Input: part model. Units: mm. Frame: model coordinates. Give positions to 0.01 mm unless a question says otherwise; leave off trailing zeros. Order: outer loops, then holes, each group sorted by start corner. A loop starts at its lowest first (then second) coordinate and runs counter-clockwise, first axis right, second up. Notation, with made-up numbers: (-25.75, 31.25) - (-5.75, 31.25) arc R7 ccw to (-5.75, 42.25) - close; hole circle Ø1 at (88.5, 82.5). An arc over 180 degrees is marked (long way). Answer in a Markdown table with one row per item. Add a question column.
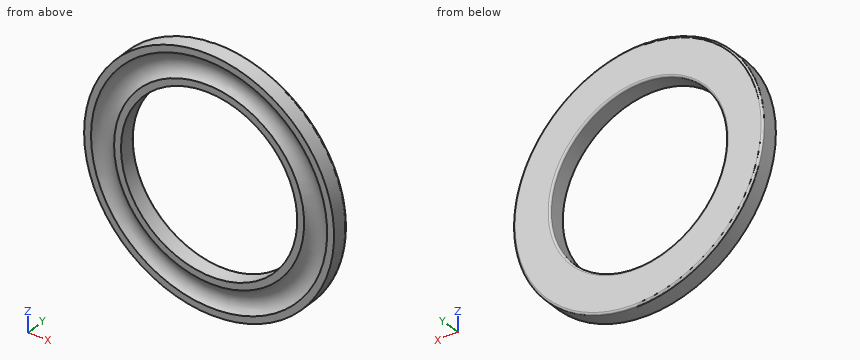
Autodesk Inventor part; units mm, degrees
ref_plane "tb_sdt_srd_XY" through (0, 0, 0) normal (0, 1, 0) x (1, 0, 0)
ref_plane "tb_sdt_srd_YZ" through (0, 0, 0) normal (1, 0, 0) x (0, 0, -1)
ref_plane "tb_sdt_srd_ZX" through (0, 0, 0) normal (0, 0, -1) x (0, 1, 0)
sketch "Sketch_1" plane through (0, 0, 0) normal (0, 0, 1) x (1, 0, 0)
  line L0 (0, 16) -> (0, 10.6667)
  line L1 (-39, 10.6667) -> (-36.8499, 10.6667)
  arc A0 (-29.6501, 10.6667) -> (-36.8499, 10.6667) centre (-33.25, 8) ccw
  line L2 (-29.6501, 10.6667) -> (-27.5, 10.6667)
  line L3 (-27.5, 10.6667) -> (-27.5, 15.4)
  arc A1 (-27.5, 15.4) -> (-28.1, 16) centre (-28.1, 15.4) ccw
  line L4 (-28.1, 16) -> (-38.4, 16)
  arc A2 (-38.4, 16) -> (-39, 15.4) centre (-38.4, 15.4) ccw
  line L5 (-39, 15.4) -> (-39, 10.6667)
revolve "Revolution1" add sketch "Sketch_1" angle 360 about axis through (0, 16, 0) along (0, 1, 0)
ref_plane "tb_sdt_srd_XY" through (0, 0, 0) normal (0, 1, 0) x (1, 0, 0)
ref_plane "tb_sdt_srd_YZ" through (0, 0, 0) normal (1, 0, 0) x (0, 0, -1)
ref_plane "tb_sdt_srd_ZX" through (0, 0, 0) normal (0, 0, -1) x (0, 1, 0)
ref_plane "tb_sdt_srd1_1_XY" through (0, 8, -33.25) normal (0, 1, 0) x (1, 0, 0)
ref_plane "tb_sdt_srd1_1_YZ" through (0, 8, -33.25) normal (1, 0, 0) x (0, 0, -1)
ref_plane "tb_sdt_srd1_1_ZX" through (0, 8, -33.25) normal (0, 0, -1) x (0, 1, 0)
ref_plane "tb_sdt_srd1_10_XY" through (25.9959, 8, 20.731) normal (0, 1, 0) x (1, 0, 0)
ref_plane "tb_sdt_srd1_10_YZ" through (25.9959, 8, 20.731) normal (1, 0, 0) x (0, 0, -1)
ref_plane "tb_sdt_srd1_10_ZX" through (25.9959, 8, 20.731) normal (0, 0, -1) x (0, 1, 0)
ref_plane "tb_sdt_srd1_11_XY" through (32.4164, 8, 7.3988) normal (0, 1, 0) x (1, 0, 0)
ref_plane "tb_sdt_srd1_11_YZ" through (32.4164, 8, 7.3988) normal (1, 0, 0) x (0, 0, -1)
ref_plane "tb_sdt_srd1_11_ZX" through (32.4164, 8, 7.3988) normal (0, 0, -1) x (0, 1, 0)
ref_plane "tb_sdt_srd1_12_XY" through (32.4164, 8, -7.3988) normal (0, 1, 0) x (1, 0, 0)
ref_plane "tb_sdt_srd1_12_YZ" through (32.4164, 8, -7.3988) normal (1, 0, 0) x (0, 0, -1)
ref_plane "tb_sdt_srd1_12_ZX" through (32.4164, 8, -7.3988) normal (0, 0, -1) x (0, 1, 0)
ref_plane "tb_sdt_srd1_13_XY" through (25.9959, 8, -20.731) normal (0, 1, 0) x (1, 0, 0)
ref_plane "tb_sdt_srd1_13_YZ" through (25.9959, 8, -20.731) normal (1, 0, 0) x (0, 0, -1)
ref_plane "tb_sdt_srd1_13_ZX" through (25.9959, 8, -20.731) normal (0, 0, -1) x (0, 1, 0)
ref_plane "tb_sdt_srd1_14_XY" through (14.4266, 8, -29.9572) normal (0, 1, 0) x (1, 0, 0)
ref_plane "tb_sdt_srd1_14_YZ" through (14.4266, 8, -29.9572) normal (1, 0, 0) x (0, 0, -1)
ref_plane "tb_sdt_srd1_14_ZX" through (14.4266, 8, -29.9572) normal (0, 0, -1) x (0, 1, 0)
ref_plane "tb_sdt_srd1_2_XY" through (-14.4266, 8, -29.9572) normal (0, 1, 0) x (1, 0, 0)
ref_plane "tb_sdt_srd1_2_YZ" through (-14.4266, 8, -29.9572) normal (1, 0, 0) x (0, 0, -1)
ref_plane "tb_sdt_srd1_2_ZX" through (-14.4266, 8, -29.9572) normal (0, 0, -1) x (0, 1, 0)
ref_plane "tb_sdt_srd1_3_XY" through (-25.9959, 8, -20.731) normal (0, 1, 0) x (1, 0, 0)
ref_plane "tb_sdt_srd1_3_YZ" through (-25.9959, 8, -20.731) normal (1, 0, 0) x (0, 0, -1)
ref_plane "tb_sdt_srd1_3_ZX" through (-25.9959, 8, -20.731) normal (0, 0, -1) x (0, 1, 0)
ref_plane "tb_sdt_srd1_4_XY" through (-32.4164, 8, -7.3988) normal (0, 1, 0) x (1, 0, 0)
ref_plane "tb_sdt_srd1_4_YZ" through (-32.4164, 8, -7.3988) normal (1, 0, 0) x (0, 0, -1)
ref_plane "tb_sdt_srd1_4_ZX" through (-32.4164, 8, -7.3988) normal (0, 0, -1) x (0, 1, 0)
ref_plane "tb_sdt_srd1_5_XY" through (-32.4164, 8, 7.3988) normal (0, 1, 0) x (1, 0, 0)
ref_plane "tb_sdt_srd1_5_YZ" through (-32.4164, 8, 7.3988) normal (1, 0, 0) x (0, 0, -1)
ref_plane "tb_sdt_srd1_5_ZX" through (-32.4164, 8, 7.3988) normal (0, 0, -1) x (0, 1, 0)
ref_plane "tb_sdt_srd1_6_XY" through (-25.9959, 8, 20.731) normal (0, 1, 0) x (1, 0, 0)
ref_plane "tb_sdt_srd1_6_YZ" through (-25.9959, 8, 20.731) normal (1, 0, 0) x (0, 0, -1)
ref_plane "tb_sdt_srd1_6_ZX" through (-25.9959, 8, 20.731) normal (0, 0, -1) x (0, 1, 0)
ref_plane "tb_sdt_srd1_7_XY" through (-14.4266, 8, 29.9572) normal (0, 1, 0) x (1, 0, 0)
ref_plane "tb_sdt_srd1_7_YZ" through (-14.4266, 8, 29.9572) normal (1, 0, 0) x (0, 0, -1)
ref_plane "tb_sdt_srd1_7_ZX" through (-14.4266, 8, 29.9572) normal (0, 0, -1) x (0, 1, 0)
ref_plane "tb_sdt_srd1_8_XY" through (0, 8, 33.25) normal (0, 1, 0) x (1, 0, 0)
ref_plane "tb_sdt_srd1_8_YZ" through (0, 8, 33.25) normal (1, 0, 0) x (0, 0, -1)
ref_plane "tb_sdt_srd1_8_ZX" through (0, 8, 33.25) normal (0, 0, -1) x (0, 1, 0)
ref_plane "tb_sdt_srd1_9_XY" through (14.4266, 8, 29.9572) normal (0, 1, 0) x (1, 0, 0)
ref_plane "tb_sdt_srd1_9_YZ" through (14.4266, 8, 29.9572) normal (1, 0, 0) x (0, 0, -1)
ref_plane "tb_sdt_srd1_9_ZX" through (14.4266, 8, 29.9572) normal (0, 0, -1) x (0, 1, 0)
properties part number "51111 Shaft raceway disc"
Q1. Section A-A, the plane x = 0. Return loops of the section in (y, z), then the cut area to 3 significant figures.
Q2. Contact query for flat-ended pins moving along their axis: P1, Ø1, axis at x = 29, y = 15, coming from the -Z side; P2, Ø1, axis at x = -29, y = 13, coming from the +Z side; P3, Ø1.5, axis at x = -6.5, y = 13.5, coming from the +Z side. Output: stop coordinate, or through.
Q3. Section C-C, the plane y = 13.6. Return loops of the section in (x, z).
Q4. Section B-B, the plane z = 0. Return loops of the section in (x, y).
Q5. Line query: probe 1 along X at (y, z) = (11.15, 21); probe 2 along Y at (x, z) = (30.5, 14); probe 3 along Z at (x, y) = (-2.5, 14.65). Output: solid intervals per line, ascending.
Computed:
| question | item | result |
|---|---|---|
| 1 | outline | (10.67, -39) - (15.4, -39) arc R0.6 ccw to (16, -38.4) - (16, -28.1) arc R0.6 ccw to (15.4, -27.5) - (10.67, -27.5) - (10.67, -29.65) arc R4.48 cw to (10.67, -36.85) - close; (10.67, 27.5) - (15.4, 27.5) arc R0.6 ccw to (16, 28.1) - (16, 38.4) arc R0.6 ccw to (15.4, 39) - (10.67, 39) - (10.67, 36.85) arc R4.48 cw to (10.67, 29.65) - close |
| 1 | area | 104 mm^2 |
| 2 | P1 | stops at z = -26.62 |
| 2 | P2 | stops at z = 26.62 |
| 2 | P3 | stops at z = 38.57 |
| 3 | outline | circle Ø78 at (0, 0); hole circle Ø55 at (0, 0) |
| 4 | outline | (-39, 10.67) - (-36.85, 10.67) arc R4.48 cw to (-29.65, 10.67) - (-27.5, 10.67) - (-27.5, 15.4) arc R0.6 ccw to (-28.1, 16) - (-38.4, 16) arc R0.6 ccw to (-39, 15.4) - close; (27.5, 10.67) - (29.65, 10.67) arc R4.48 cw to (36.85, 10.67) - (39, 10.67) - (39, 15.4) arc R0.6 ccw to (38.4, 16) - (28.1, 16) arc R0.6 ccw to (27.5, 15.4) - close |
| 5 | probe 1 | x = -32.86 to -29.78, -21.51 to -17.76, 17.76 to 21.51, 29.78 to 32.86 |
| 5 | probe 2 | y = 12.47 to 16 |
| 5 | probe 3 | z = -38.92 to -27.39, 27.39 to 38.92 |
